For this review, take the finished solid that the model builds, in its own axes (mm). A direction names the side the tool comes from. Round coordinates to 2 decimals unless told otherwise and drop trailing zeros. Loops run counter-clockwise (first coordinate to the right, second up) from the corner with the lowest first, then second, coordinate; pieces in that order, holes last. Notation, with made-up numbers: (19, 64.5) -> (33, 64.5) arc R22 ccw to (33, 82.5) -> close; hole circle Ø6 at (47.25, 8). An arc over 180 degrees is marked (long way). Write each question's results on one line, items separated by ' | '.
```python
from build123d import *

# Parameters (mm, degrees)
F0_W     = 10
F0_H     = 16
F1_DEPTH = 2
F2_W     = 8
F2_H     = 2
F2_W_2   = 2
F2_H_2   = 3
F3_DEPTH = 2


with BuildPart() as f1:
    # F0 (on Top) → F1 (new body)
    with BuildSketch(Plane.XY):
        Rectangle(F0_W, F0_H)
    extrude(amount=F1_DEPTH)

    # F2 (on face) → F3 (join)
    with BuildSketch(Plane.XY.offset(2)):
        Rectangle(F2_W, F2_H)
        with Locations((0, -6)):
            Rectangle(F2_W, F2_H)
        with Locations((-3, 3)):
            Rectangle(F2_W_2, F2_H_2)
        with Locations((3, 3)):
            Rectangle(F2_W_2, F2_H_2)
        with Locations((-3, -3)):
            Rectangle(F2_W_2, F2_H_2)
        with Locations((3, -3)):
            Rectangle(F2_W_2, F2_H_2)
        with Locations((0, 6)):
            Rectangle(F2_W, F2_H)
    extrude(amount=F3_DEPTH)


solid = f1.part
```
1. Consider section C-C (x = 3.25). State the section outline as (y, z) points, plus the area to 3 significant figures.
Values found:
outline: (-8, 0) -> (8, 0) -> (8, 2) -> (7, 2) -> (7, 4) -> (5, 4) -> (5, 2) -> (4.5, 2) -> (4.5, 4) -> (1.5, 4) -> (1.5, 2) -> (1, 2) -> (1, 4) -> (-1, 4) -> (-1, 2) -> (-1.5, 2) -> (-1.5, 4) -> (-4.5, 4) -> (-4.5, 2) -> (-5, 2) -> (-5, 4) -> (-7, 4) -> (-7, 2) -> (-8, 2) -> close | area: 56.0 mm2
2. Consider section A-A (z = 3.4). State the section outline as (x, y) points, plus the area to 3 significant figures.
Values found:
outline: (-4, -7) -> (4, -7) -> (4, -5) -> (-4, -5) -> close; (-4, -4.5) -> (-2, -4.5) -> (-2, -1.5) -> (-4, -1.5) -> close; (-4, -1) -> (4, -1) -> (4, 1) -> (-4, 1) -> close; (-4, 1.5) -> (-2, 1.5) -> (-2, 4.5) -> (-4, 4.5) -> close; (-4, 5) -> (4, 5) -> (4, 7) -> (-4, 7) -> close; (2, -4.5) -> (4, -4.5) -> (4, -1.5) -> (2, -1.5) -> close; (2, 1.5) -> (4, 1.5) -> (4, 4.5) -> (2, 4.5) -> close | area: 72.0 mm2
3. Consider section B-B (y = 3.5). State the section outline as (x, z) points.
Values found:
outline: (-5, 0) -> (5, 0) -> (5, 2) -> (4, 2) -> (4, 4) -> (2, 4) -> (2, 2) -> (-2, 2) -> (-2, 4) -> (-4, 4) -> (-4, 2) -> (-5, 2) -> close
4. For pin 1 (1.6 mm diameter, centred on y = 6, z = 3.5, fed in from -X); pin 2 (1 mm diameter, centred on x = -3, z = 3, fed in from +Y); pin 3 (1 mm diameter, centred on y = 0.5, z = 3.5, fed in from +X), all flat-tipped, find the tip position at first contact; note any pin that passes through.
Values found:
pin 1: stops at x = -4 | pin 2: stops at y = 7 | pin 3: stops at x = 4
5. Consider section D-D (x = 0.75). State the section outline as (y, z) points, plus the area to 3 significant figures.
Values found:
outline: (-8, 0) -> (8, 0) -> (8, 2) -> (7, 2) -> (7, 4) -> (5, 4) -> (5, 2) -> (1, 2) -> (1, 4) -> (-1, 4) -> (-1, 2) -> (-5, 2) -> (-5, 4) -> (-7, 4) -> (-7, 2) -> (-8, 2) -> close | area: 44.0 mm2
6. To check wall thickness, follow probe 1 along Y at (x, z) = (-0.5, 2.45); probe 2 along Y at (x, z) = (2.5, 2.6); probe 3 along X at (y, z) = (-3.5, 2.3). State the ranges of each line that lie inside material, in increasing order.
Values found:
probe 1: y = -7 to -5, -1 to 1, 5 to 7 | probe 2: y = -7 to -5, -4.5 to -1.5, -1 to 1, 1.5 to 4.5, 5 to 7 | probe 3: x = -4 to -2, 2 to 4
7. Draft analysis for pull direction Y (two halves, no side actions). For faces 5 (the face through (2, 3, 3)), 6 (the face through (-3, 3, 4)), state which applies: released by +Y, released by -Y, zero draft, split by the parting line, or undercut.
Values found:
face 5: undercut | face 6: zero draft
8. Tool access review of faces 1 (the face through (0, 5, 3)), 2 (the face through (-4, 6, 3)), 3 (the face through (4, 3, 3)), 4 (the face through (-5, 0, 1)): name each direction out of +Z, -Z, +X, -X, +Y, -Y from which nothing blocks a thin tool from reaching the whole face with its end or side.
Values found:
face 1: +Z, +X, -X | face 2: +Z, -X, +Y, -Y | face 3: +Z, +X, +Y, -Y | face 4: +Z, -Z, -X, +Y, -Y
